Source: CAD feature listing. Evaluate the final solid. Frame: model axes, mm. Face numbers are marked on the shaded views. A direction names the side the tool comes from. Round coordinates to 2 decimals unless told otherwise and drop trailing zeros. Write each loop counter-clockwise with the first axis right and the second up, starting at its lowest first coordinate (ties: lowest second). Pieces come first, ordered by that corner, then holes. Notation, with made-up numbers: M -29.75,48.25 L -8.75,48.25 A11 ccw -8.75,65.25 Z; hole C -30.5,-28.75 d4. An arc over 180 degrees is marked long. Answer in a Markdown table with one row per item. Add a question column.
Item 1: Material intervals for probe 1 along Z at (x, y) = (0, 4.5); probe 2 along X at (y, z) = (6, 0); probe 3 along X at (y, z) = (0.7, 0), sorted ascending.
Item 2: Contact query for flat-ended pins moving along their axis: pin 1 (1.9 mm diameter, centred on x = 0.5, z = -0.5, fed in from -Y); pin 2 (1 mm diameter, centred on y = 12, z = -23, fed in from -X); pin 3 (2 mm diameter, centred on x = -4.5, y = 11.5, fed in from -Z). Output: stop coordinate, or through.
Item 3: Cut plane A-A on y = 24. Return loops of the section in (x, z).
Item 4: Set-up query: the marked faces 1, 2 and 3. Return all of +Z, -Z, +X, -X, +Y, -Y with unobstructed straight access to the full face (end or side cutting, diameter ignored); none if empty.
Item 5: Cut plane C-C on y = 29. Return loops of the section in (x, z).
Item 6: Cut plane B-B on z = -9.5. Return loops of the section in (x, y), and give its area (3 significant figures).
Item 7: Cut plane D-D on z = 0. Return loops of the section in (x, y).
Item 8: Mould query, pull axis Y, two halves, no side actions, for the marked faces 4, 5 and 6. Classes: released by +Y, released by -Y, zero draft, split by the parting line, or undercut.
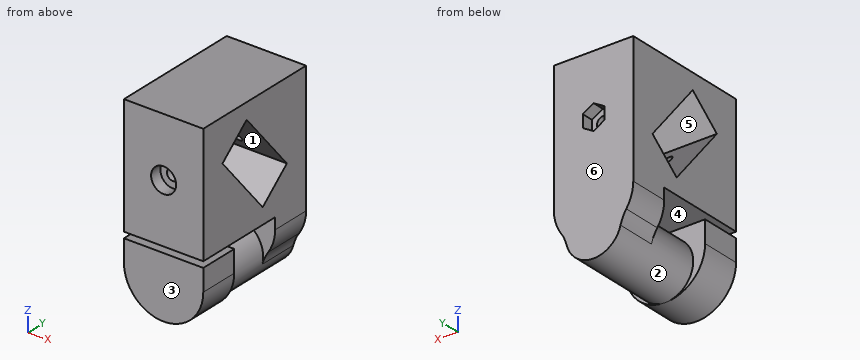
from build123d import *

# Parameters (mm, degrees)
SKETCH_1_W                      = 20
SKETCH_1_H                      = 30
EXTRUDE_1_DEPTH                 = 33.2
SKETCH_2_R                      = 1.5
CUT_EXTRUDE_1_DEPTH             = 38.778830051
CUT_EXTRUDE_4_DEPTH             = 30
SKETCH1_W                       = 20
SKETCH1_H                       = 10
BOSS_EXTRUDE2_DEPTH             = 10
BOSS_EXTRUDE3_REACH             = 37.542
SKETCH2_R                       = 7
BOSS_EXTRUDE3_DIRECTION_2_REACH = 37.542
FILLET1_R                       = 10
SKETCH3_W                       = 20
SKETCH3_H                       = 15.5
BOSS_EXTRUDE4_DEPTH             = 10
FILLET2_R                       = 10
SKETCH4_R                       = 3.15
CUT_EXTRUDE1_DEPTH              = 3
CUT_EXTRUDE2_DEPTH              = 3


with BuildPart() as part:
    # Эскиз1 → Бобышка-Вытянуть1 (new body)
    with BuildSketch(Plane(origin=(0, 0, 0), x_dir=(1, 0, 0), z_dir=(0, 1, 0))):
        Rectangle(SKETCH_1_W, SKETCH_1_H)
    extrude(amount=EXTRUDE_1_DEPTH)

    # Эскиз2 → Вырез-Вытянуть1 (cut, through all)
    with BuildSketch(Plane(origin=(0, 33.2, 0), x_dir=(1, 0, 0), z_dir=(0, 1, 0))):
        with Locations(Location((0, 0, 0), (0, 0, 270))):
            Circle(SKETCH_2_R)
    extrude(amount=-CUT_EXTRUDE_1_DEPTH, mode=Mode.SUBTRACT)

    # Эскиз5 → Вырез-Вытянуть4 (cut)
    with BuildSketch(Plane.ZY.offset(10)):
        Polygon((-4.458832066, 26.998981518), (-11.015265685, 19.185328198), (4.458832066, 6.201018482), (11.015265685, 14.014671802), align=None)
    extrude(amount=-CUT_EXTRUDE_4_DEPTH, mode=Mode.SUBTRACT)

    # Sketch1 → Boss-Extrude2 (add)
    with BuildSketch(Plane(origin=(0, 0, -15), x_dir=(-1, 0, 0), z_dir=(0, 0, -1))):
        with Locations((0, 28.2)):
            Rectangle(SKETCH1_W, SKETCH1_H)
    extrude(amount=BOSS_EXTRUDE2_DEPTH)

    # Boss-Extrude3: up to this face of the body (flat: up to its plane)
    boss_extrude3_end = Plane(part.part.faces().sort_by_distance((0, 0, 14.639444872))[0])
    # Sketch2 → Boss-Extrude3 (add, up to the picked face)
    with BuildSketch(Plane.XZ.offset(-23.2), mode=Mode.PRIVATE) as boss_extrude3_sk1:
        with Locations((0, -25)):
            Circle(SKETCH2_R)
    boss_extrude3_tool1 = split(extrude(boss_extrude3_sk1.sketch, amount=BOSS_EXTRUDE3_REACH, mode=Mode.PRIVATE), bisect_by=boss_extrude3_end, keep=Keep.BOTH, mode=Mode.PRIVATE)
    add(boss_extrude3_tool1.solids().sort_by(Axis((0, 23.2, -25), (0, -1, 0)))[0])

    # Boss-Extrude3 direction 2: up to this face of the body (flat: up to its plane)
    boss_extrude3_direction_2_end = Plane(part.part.faces().sort_by_distance((0, 33.2, -5.044572477))[0])
    # Sketch2 → Boss-Extrude3 direction 2 (add, up to the picked face)
    with BuildSketch(Plane.XZ.offset(-23.2), mode=Mode.PRIVATE) as boss_extrude3_direction_2_sk1:
        with Locations((0, -25)):
            Circle(SKETCH2_R)
    boss_extrude3_direction_2_tool1 = split(extrude(boss_extrude3_direction_2_sk1.sketch, amount=-BOSS_EXTRUDE3_DIRECTION_2_REACH, mode=Mode.PRIVATE), bisect_by=boss_extrude3_direction_2_end, keep=Keep.BOTH, mode=Mode.PRIVATE)
    add(boss_extrude3_direction_2_tool1.solids().sort_by(Axis((0, 23.2, -25), (0, 1, 0)))[0])

    # Fillet1
    # the kernel refuses this fillet: 10 mm, written as the material it takes off along each edge
    with BuildSketch(Plane(origin=(-10, 5.346428929, -25), x_dir=(0, 0, 1), z_dir=(0, 1, 0)), Plane(origin=(10, 51.053571071, -25), x_dir=(0, 0, 1), z_dir=(0, -1, 0))) as fillet1_piece_1:
        with BuildLine():
            CenterArc((7.141428429, 10), FILLET1_R, 224.427004001, 45.572995999)
            Line((0, 3), (-0.142828569, 2.86))
            ThreePointArc((-0.142828569, 2.86), (-0.2, 1.5), (-0.2, 0))
            Line((-0.2, 0), (0, -0.2))
            Line((0, -0.2), (7.141428429, -0.2))
            Line((7.141428429, -0.2), (7.141428429, 0))
        make_face()
    extrude(amount=45.707142143, mode=Mode.SUBTRACT)

    # Sketch3 → Boss-Extrude4 (add)
    with BuildSketch(Plane.XZ):
        with Locations((0, -24.25)):
            Rectangle(SKETCH3_W, SKETCH3_H)
    extrude(amount=-BOSS_EXTRUDE4_DEPTH)

    # Fillet2
    # the kernel refuses this fillet: 10 mm, written as the material it adds along each edge
    with BuildSketch(Plane(origin=(7, 23.2, -25), x_dir=(0.6436039974439222, 0, 0.7653586704769234), z_dir=(0, 1, 0))) as fillet2_piece_1:
        with BuildLine():
            CenterArc((2.881578556, 9.953762577), FILLET2_R, 244.245370549, 20.242721963)
            ThreePointArc((-1.463601761, 0.947131242), (-0.702200702, 0.519306771), (0, 0))
            ThreePointArc((0, 0), (0.960526185, 0.046237423), (1.921052371, 0))
        make_face()
    extrude(amount=10)
    with BuildSketch(Plane(origin=(-7, 33.2, -25), x_dir=(0.12452332997196464, 0, -0.9922166801121081), z_dir=(0, -1, 0))) as fillet2_piece_2:
        with BuildLine():
            CenterArc((2.988559919, -9.922166801), FILLET2_R, 97.153229531, 20.242721963)
            ThreePointArc((-1.612810589, -1.043687796), (-0.781284983, -0.560662311), (0, 0))
            ThreePointArc((0, 0), (0.87166331, -0.054483239), (1.74332662, 0))
        make_face()
    extrude(amount=10)
    # the kernel refuses this fillet: 10 mm, written as the material it takes off along each edge
    with BuildSketch(Plane(origin=(10, -25, -32), x_dir=(0, 0, 1), z_dir=(0, 1, 0)), Plane(origin=(-10, -25, -32), x_dir=(1, 0, 0), z_dir=(0, 1, 0))) as fillet2_2_piece_1:
        with BuildLine():
            CenterArc((FILLET2_R, -FILLET2_R), FILLET2_R, 90, 90)
            Line((0, -FILLET2_R), (0, 0))
            Line((0, 0), (FILLET2_R, 0))
        make_face()
    extrude(amount=60, mode=Mode.SUBTRACT)

    # Sketch4 → Cut-Extrude1 (cut)
    with BuildSketch(Plane.XZ):
        with Locations(Location((0, 0, 0), (0, 0, 270))):
            Circle(SKETCH4_R)
    extrude(amount=-CUT_EXTRUDE1_DEPTH, mode=Mode.SUBTRACT)

    # Sketch5 → Cut-Extrude2 (cut)
    with BuildSketch(Plane(origin=(0, 33.2, 0), x_dir=(1, 0, 0), z_dir=(0, 1, 0))):
        Polygon((0, 3.15), (-2.727980022, 1.575), (-2.727980022, -1.575), (0, -3.15), (2.727980022, -1.575), (2.727980022, 1.575), align=None)
    extrude(amount=-CUT_EXTRUDE2_DEPTH, mode=Mode.SUBTRACT)


solid = part.part
Results below:
| question | item | result |
|---|---|---|
| 1 | probe 1 | -32 to -16.5, -15 to -1.5, 1.5 to 15 |
| 1 | probe 2 | -10 to -1.5, 1.5 to 10 |
| 1 | probe 3 | -10 to -3.15, 3.15 to 10 |
| 2 | pin 1 | y = 3 |
| 2 | pin 2 | x = -6.84 |
| 2 | pin 3 | z = -31.06 |
| 3 | outline | M -10,-17.86 A10 ccw -8.24,-23.53 A10 cw -6.78,-26.73 A7 ccw 6.78,-26.73 A10 cw 8.24,-23.53 A10 ccw 10,-17.86 L 10,-6.98 L -10,-6.98 Z; M -10,-0.88 L -1.21,-0.88 A1.5 cw long 1.21,-0.88 L 10,-0.88 L 10,15 L -10,15 Z |
| 4 | face 1 | +X, -X |
| 4 | face 2 | none |
| 4 | face 3 | +Z, -Z, +X, -X, -Y |
| 5 | outline | M -10,-17.86 A10 ccw -8.24,-23.53 A10 cw -6.78,-26.73 A7 ccw 6.78,-26.73 A10 cw 8.24,-23.53 A10 ccw 10,-17.86 L 10,15 L -10,15 Z; hole C 0,0 d3 |
| 6 | outline | M -10,0 L 10,0 L 10,17.91 L -10,17.91 Z; M -10,20.99 L 10,20.99 L 10,33.2 L -10,33.2 Z |
| 6 | area | 602 mm2 |
| 7 | outline | M -10,0 L -3.15,0 L -3.15,3 L -1.5,3 L -1.5,9.94 L -10,9.94 Z; M -10,23.26 L -1.5,23.26 L -1.5,30.2 L -2.73,30.2 L -2.73,33.2 L -10,33.2 Z; M 1.5,3 L 3.15,3 L 3.15,0 L 10,0 L 10,9.94 L 1.5,9.94 Z; M 1.5,23.26 L 10,23.26 L 10,33.2 L 2.73,33.2 L 2.73,30.2 L 1.5,30.2 Z |
| 8 | face 4 | zero draft |
| 8 | face 5 | undercut |
| 8 | face 6 | released by +Y |
